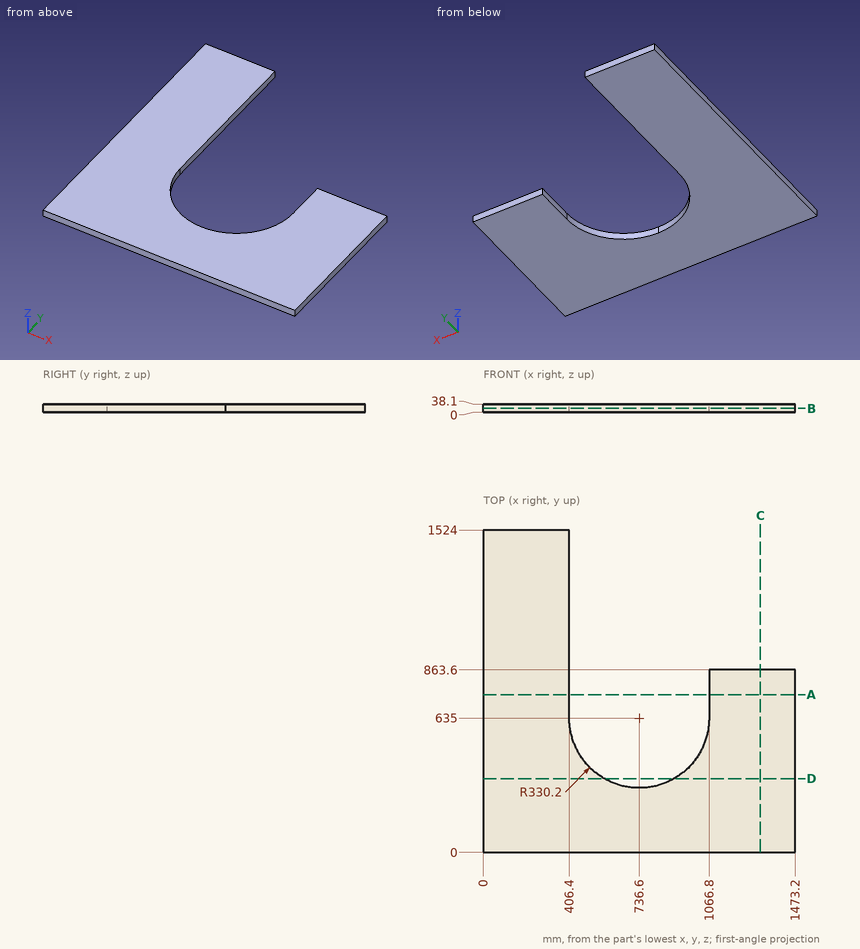
Part print with two shaded views. Sizes in mm from the minimum x, y, z corner. Round coordinates to 2 decimals unless told otherwise and drop trailing zeros. Write each loop counter-clockwise with the first axis right and the second up, starting at its lowest first coordinate (ties: lowest second). Pieces come first, ordered by that corner, then holes. Notation, with made-up numbers: (-15, 56) - (40, 56) arc R23 cw to (40, 85) - close; hole circle Ø8 at (-4.75, -37.5). An arc over 180 degrees is marked (long way). Use CSV: the item, a comma, the result in double quotes.
Item 1: Slice it at D-D, the plane y = 348.5. Write the cut outline in (x, z).
Results list:
outline,"(0, 0) - (572.44, 0) - (572.44, 38.1) - (0, 38.1) - close; (900.76, 0) - (1473.2, 0) - (1473.2, 38.1) - (900.76, 38.1) - close"
Item 2: Slice it at B-B, the plane z = 17. Write the cut outline in (x, y).
Results list:
outline,"(0, 0) - (1473.2, 0) - (1473.2, 863.6) - (1066.8, 863.6) - (1066.8, 635) arc R330.2 cw to (736.6, 304.8) arc R330.2 cw to (406.4, 635) - (406.4, 1524) - (0, 1524) - close"
Item 3: Wall check: L1, parallel to X at y = 848.5, z = 19.5; L2, parallel to Y at x = 1412, z = 2.5; L3, parallel to X at y = 510.5, z = 24.5. Give the ranges that are in metal, low to high.
Results list:
L1,"x = 0 to 406.4, 1066.8 to 1473.2"
L2,"y = 0 to 863.6"
L3,"x = 0 to 430.77, 1042.43 to 1473.2"
Item 4: Slice it at C-C, the plane x = 1310. Write the cut outline in (y, z).
Results list:
outline,"(0, 0) - (863.6, 0) - (863.6, 38.1) - (0, 38.1) - close"
Item 5: Slice it at A-A, the plane y = 746.5. Write the cut outline in (x, z).
Results list:
outline,"(0, 0) - (406.4, 0) - (406.4, 38.1) - (0, 38.1) - close; (1066.8, 0) - (1473.2, 0) - (1473.2, 38.1) - (1066.8, 38.1) - close"
